```python
from build123d import *
from build123d.topology import SkipClean

# Parameters (mm, degrees)
SKETCH1_W            = 220
SKETCH1_H            = 40
SKETCH1_R            = 6
SKETCH1_R_2          = 1.7
SKETCH1_R_3          = 11
BOSS_EXTRUDE1_DEPTH  = 10
BOSS_EXTRUDE3_START  = -20
SKETCH3_R            = 9.05
SKETCH3_R_2          = 6
BOSS_EXTRUDE3_DEPTH  = 20
SKETCH4_W            = 50
SKETCH4_H            = 65
BOSS_EXTRUDE4_DEPTH  = 10
SKETCH5_W            = 57.5
SKETCH5_H            = 8.5
BOSS_EXTRUDE5_DEPTH  = 20
CUT_EXTRUDE3_START   = -40
SKETCH7_W            = 23
SKETCH7_H            = 15.765385727
CUT_EXTRUDE3_DEPTH   = 40
SKETCH11_W           = 10
SKETCH11_H           = 20
BOSS_EXTRUDE6_DEPTH  = 10
SKETCH12_W           = 10
SKETCH12_H           = 20
BOSS_EXTRUDE7_DEPTH  = 10
FILLET2_R            = 3
FILLET3_R            = 10
BOSS_EXTRUDE8_START  = 10
BOSS_EXTRUDE8_DEPTH  = 10
SKETCH20_R           = 2.15
CUT_EXTRUDE11_DEPTH  = 277
SKETCH19_R           = 2.15
CUT_EXTRUDE12_DEPTH  = 270
BOSS_EXTRUDE9_DEPTH  = 10
SKETCH22_W           = 40
SKETCH22_H           = 40
BOSS_EXTRUDE10_DEPTH = 31.75
SKETCH23_W           = 30.8
SKETCH23_H           = 25.6
CUT_EXTRUDE13_DEPTH  = 263.144
SKETCH24_R           = 4.65
CUT_EXTRUDE14_DEPTH  = 48.144
FILLET4_R            = 3
SKETCH25_R           = 1.7
CUT_EXTRUDE16_DEPTH  = 60.144


with BuildPart() as part:
    # Sketch1 → Boss-Extrude1 (new body)
    with BuildSketch(Plane.XY):
        with Locations((1.5, 0)):
            Rectangle(SKETCH1_W, SKETCH1_H)
        with Locations((99, 0)):
            Circle(SKETCH1_R, mode=Mode.SUBTRACT)
        with Locations((-96, 0)):
            Circle(SKETCH1_R, mode=Mode.SUBTRACT)
        with Locations((-15.5, 15.5)):
            Circle(SKETCH1_R_2, mode=Mode.SUBTRACT)
        with Locations((15.5, 15.5)):
            Circle(SKETCH1_R_2, mode=Mode.SUBTRACT)
        Circle(SKETCH1_R_3, mode=Mode.SUBTRACT)
        with Locations((-15.5, -15.5)):
            Circle(SKETCH1_R_2, mode=Mode.SUBTRACT)
        with Locations((15.5, -15.5)):
            Circle(SKETCH1_R_2, mode=Mode.SUBTRACT)
        with Locations((75, 0)):
            Circle(SKETCH1_R_3, mode=Mode.SUBTRACT)
        with Locations((59.5, 15.5)):
            Circle(SKETCH1_R_2, mode=Mode.SUBTRACT)
        with Locations((59.5, -15.5)):
            Circle(SKETCH1_R_2, mode=Mode.SUBTRACT)
        with Locations((90.5, 15.5)):
            Circle(SKETCH1_R_2, mode=Mode.SUBTRACT)
        with Locations((90.5, -15.5)):
            Circle(SKETCH1_R_2, mode=Mode.SUBTRACT)
    extrude(amount=BOSS_EXTRUDE1_DEPTH)

    # Sketch3 → Boss-Extrude3 (add)
    # profile 1 of 2: a face of its own
    with BuildSketch(Plane.XY.offset(10).offset(BOSS_EXTRUDE3_START)):
        with Locations((-96, 0)):
            Circle(SKETCH3_R)
        with Locations((-96, 0)):
            Circle(SKETCH3_R_2, mode=Mode.SUBTRACT)
    # profile 2 of 2: a face of its own
    with BuildSketch(Plane.XY.offset(10).offset(BOSS_EXTRUDE3_START)):
        with Locations((99, 0)):
            Circle(SKETCH3_R)
        with Locations((99, 0)):
            Circle(SKETCH3_R_2, mode=Mode.SUBTRACT)
    extrude(amount=BOSS_EXTRUDE3_DEPTH)

    # Sketch4 → Boss-Extrude4 (add)
    with BuildSketch(Plane(origin=(111.5, 0, 0), x_dir=(0, 0, -1), z_dir=(1, 0, 0))):
        with Locations((15, 0)):
            Rectangle(SKETCH4_W, SKETCH4_H)
    extrude(amount=BOSS_EXTRUDE4_DEPTH)

    # Sketch5 → Boss-Extrude5 (add)
    with BuildSketch(Plane(origin=(0, 0, 0), x_dir=(-1, 0, 0), z_dir=(0, 0, -1))):
        with Locations((-82.75, 15.75)):
            Rectangle(SKETCH5_W, SKETCH5_H)
        with Locations((-82.75, -15.75)):
            Rectangle(SKETCH5_W, SKETCH5_H)
    extrude(amount=BOSS_EXTRUDE5_DEPTH)

    # Sketch7 → Cut-Extrude3 (cut)
    with BuildSketch(Plane(origin=(0, 20, 0), x_dir=(1, 0, 0), z_dir=(0, 1, 0)).offset(CUT_EXTRUDE3_START)):
        with Locations((72.5, 7.882692864)):
            Rectangle(SKETCH7_W, SKETCH7_H)
    extrude(amount=CUT_EXTRUDE3_DEPTH, mode=Mode.SUBTRACT)

    # Sketch11 → Boss-Extrude6 (add)
    with BuildSketch(Plane(origin=(0, 32.5, 0), x_dir=(1, 0, 0), z_dir=(0, 1, 0))):
        with Locations((116.5, 30)):
            Rectangle(SKETCH11_W, SKETCH11_H)
    extrude(amount=BOSS_EXTRUDE6_DEPTH)

    # Sketch12 → Boss-Extrude7 (add)
    with BuildSketch(Plane.XZ.offset(32.5)):
        with Locations((116.5, -30)):
            Rectangle(SKETCH12_W, SKETCH12_H)
    extrude(amount=BOSS_EXTRUDE7_DEPTH)

    # Fillet2
    # the kernel refuses this fillet: 3 mm, written as the material it adds along each edge
    with BuildSketch(Plane(origin=(121.5, -32.5, -20), x_dir=(0, 0, 1), z_dir=(-1, 0, 0))) as fillet2_piece_1:
        with BuildLine():
            CenterArc((FILLET2_R, -FILLET2_R), FILLET2_R, 90, 90)
            Line((0, -FILLET2_R), (0, 0))
            Line((0, 0), (FILLET2_R, 0))
        make_face()
    extrude(amount=10)
    with BuildSketch(Plane(origin=(111.5, 32.5, -20), x_dir=(0, 1, 0), z_dir=(1, 0, 0))) as fillet2_piece_2:
        with BuildLine():
            CenterArc((FILLET2_R, FILLET2_R), FILLET2_R, 180, 90)
            Line((0, FILLET2_R), (0, 0))
            Line((0, 0), (FILLET2_R, 0))
        make_face()
    extrude(amount=10)
    with BuildSketch(Plane(origin=(84, 11.5, -15.765385727), x_dir=(0, 0, 1), z_dir=(0, 1, 0)), Plane(origin=(61, 11.5, -15.765385727), x_dir=(1, 0, 0), z_dir=(0, 1, 0)), Plane(origin=(84, 11.5, 0), x_dir=(-1, 0, 0), z_dir=(0, 1, 0)), Plane(origin=(84, -20, 0), x_dir=(-1, 0, 0), z_dir=(0, 1, 0))) as fillet2_piece_3:
        with BuildLine():
            CenterArc((FILLET2_R, -FILLET2_R), FILLET2_R, 90, 90)
            Line((0, -FILLET2_R), (0, 0))
            Line((0, 0), (FILLET2_R, 0))
        make_face()
    extrude(amount=8.5)
    with BuildSketch(Plane(origin=(61, 11.5, 0), x_dir=(1, 0, 0), z_dir=(0, 1, 0))) as fillet2_piece_4_section:
        with BuildLine():
            CenterArc((FILLET2_R, FILLET2_R), FILLET2_R, 180, 90)
            Line((0, FILLET2_R), (0, 0))
            Line((0, 0), (FILLET2_R, 0))
        make_face()
    fillet2_piece_4 = extrude(amount=10.7, mode=Mode.PRIVATE)
    fillet2_piece_4 = fillet2_piece_4 - Plane(origin=(59.5, 15.5, -0.653390462), x_dir=(1, 0, 0), z_dir=(0, 0, -1)) * Cylinder(1.7, 34, mode=Mode.PRIVATE)
    fillet2_piece_4 = split(fillet2_piece_4, bisect_by=Plane(origin=(61.689155884, 20, -0.653390462), z_dir=(0, -1, 0)), keep=Keep.TOP, mode=Mode.PRIVATE)
    add(fillet2_piece_4)
    with BuildSketch(Plane(origin=(84, -20, -15.765385727), x_dir=(-1, 0, 0), z_dir=(0, 1, 0))) as fillet2_piece_5:
        with BuildLine():
            CenterArc((FILLET2_R, FILLET2_R), FILLET2_R, 180, 90)
            Line((0, FILLET2_R), (0, 0))
            Line((0, 0), (FILLET2_R, 0))
        make_face()
    extrude(amount=8.5)
    # the kernel refuses this fillet: 3 mm, written as the material it takes off along each edge
    with BuildSketch(Plane(origin=(104, -32.5, 10), x_dir=(0, 0, -1), z_dir=(1, 0, 0)), Plane(origin=(129, -42.5, -20), x_dir=(0, 1, 0), z_dir=(-1, 0, 0)), Plane(origin=(129, 42.5, -40), x_dir=(0, -1, 0), z_dir=(-1, 0, 0))) as fillet2_2_piece_1:
        with BuildLine():
            CenterArc((FILLET2_R, FILLET2_R), FILLET2_R, 180, 90)
            Line((0, FILLET2_R), (0, 0))
            Line((0, 0), (FILLET2_R, 0))
        make_face()
    extrude(amount=25, mode=Mode.SUBTRACT)
    with BuildSketch(Plane(origin=(104, -42.5, -40), x_dir=(0, 0, 1), z_dir=(1, 0, 0)), Plane(origin=(104, 32.5, 10), x_dir=(0, 0, -1), z_dir=(1, 0, 0)), Plane(origin=(104, 42.5, -20), x_dir=(0, 0, -1), z_dir=(1, 0, 0))) as fillet2_2_piece_2:
        with BuildLine():
            CenterArc((FILLET2_R, -FILLET2_R), FILLET2_R, 90, 90)
            Line((0, -FILLET2_R), (0, 0))
            Line((0, 0), (FILLET2_R, 0))
        make_face()
    extrude(amount=25, mode=Mode.SUBTRACT)

    # Fillet3
    fillet3_edges = [part.edges().sort_by_distance(p)[0] for p in [
        (111.5, 15.75, -20),
        (111.5, -15.75, -20),
    ]]
    fillet(fillet3_edges, radius=FILLET3_R)

    # Sketch13 → Boss-Extrude8 (add)
    with BuildSketch(Plane.ZY.offset(108.5).offset(BOSS_EXTRUDE8_START)):
        with BuildLine():
            Line((10, 29.5), (10, -29.5))
            ThreePointArc((10, -29.5), (9.121320344, -31.621320344), (7, -32.5))
            Line((7, -32.5), (-17, -32.5))
            ThreePointArc((-17, -32.5), (-19.121320344, -33.378679656), (-20, -35.5))
            Line((-20, -35.5), (-20, -39.5))
            ThreePointArc((-20, -39.5), (-20.878679656, -41.621320344), (-23, -42.5))
            Line((-23, -42.5), (-37, -42.5))
            ThreePointArc((-37, -42.5), (-39.121320344, -41.621320344), (-40, -39.5))
            Line((-40, -39.5), (-40, 39.5))
            ThreePointArc((-40, 39.5), (-39.121320344, 41.621320344), (-37, 42.5))
            Line((-37, 42.5), (-23, 42.5))
            ThreePointArc((-23, 42.5), (-20.878679656, 41.621320344), (-20, 39.5))
            Line((-20, 39.5), (-20, 35.5))
            ThreePointArc((-20, 35.5), (-19.121320344, 33.378679656), (-17, 32.5))
            Line((-17, 32.5), (7, 32.5))
            ThreePointArc((7, 32.5), (9.121320344, 31.621320344), (10, 29.5))
        make_face()
    extrude(amount=-BOSS_EXTRUDE8_DEPTH)

    # Sketch20 → Cut-Extrude11 (cut)
    with BuildSketch(Plane.ZY.offset(118.5)):
        with Locations((-31, 31.5)):
            Circle(SKETCH20_R)
    extrude(amount=-CUT_EXTRUDE11_DEPTH, mode=Mode.SUBTRACT)

    # Sketch19 → Cut-Extrude12 (cut)
    with BuildSketch(Plane.ZY.offset(118.5)):
        with Locations((-31, -31.5)):
            Circle(SKETCH19_R)
    extrude(amount=-CUT_EXTRUDE12_DEPTH, mode=Mode.SUBTRACT)

    # Sketch16 → Boss-Extrude9 (add)
    with BuildSketch(Plane.XY.offset(10)):
        with BuildLine():
            Line((-98.5, 84), (-118.5, 84))
            Line((-118.5, 84), (-118.5, 29.5))
            Line((-118.5, 29.5), (-108.5, 29.5))
            Line((-108.5, 29.5), (-108.5, 20))
            Line((-108.5, 20), (-78.5, 20))
            ThreePointArc((-78.5, 20), (-92.297269835, 26.202730165), (-98.5, 40))
            Line((-98.5, 40), (-98.5, 84))
        make_face()
    boss_extrude9 = extrude(amount=-BOSS_EXTRUDE9_DEPTH)

    # Mirror1: Boss-Extrude9 across plane
    add(boss_extrude9.mirror(Plane(origin=(1.5, 0, 0), x_dir=(0, 0, 1), z_dir=(1, 0, 0))))

    # Sketch22 → Boss-Extrude10 (add)
    with BuildSketch(Plane(origin=(0, 84, 0), x_dir=(1, 0, 0), z_dir=(0, 1, 0))):
        with Locations((101.5, 10)):
            Rectangle(SKETCH22_W, SKETCH22_H)
    boss_extrude10 = extrude(amount=BOSS_EXTRUDE10_DEPTH)

    # Mirror2: Boss-Extrude10 across plane
    add(boss_extrude10.mirror(Plane(origin=(1.5, 0, 0), x_dir=(0, 0, 1), z_dir=(1, 0, 0))))

    # Sketch23 → Cut-Extrude13 (cut)
    with BuildSketch(Plane.ZY.offset(118.5)):
        with Locations((-10, 102.95)):
            Rectangle(SKETCH23_W, SKETCH23_H)
    extrude(amount=-CUT_EXTRUDE13_DEPTH, mode=Mode.SUBTRACT)

    # Sketch24 → Cut-Extrude14 (cut)
    with BuildSketch(Plane.XZ.offset(-84)):
        with Locations((-98.5, -10)):
            Circle(SKETCH24_R)
        with Locations((101.5, -10)):
            Circle(SKETCH24_R)
    extrude(amount=-CUT_EXTRUDE14_DEPTH, mode=Mode.SUBTRACT)

    # Fillet4
    fillet4_edges = [part.edges().sort_by_distance(p)[0] for p in [
        (-98.5, 84, 5),
        (-108.5, 84, 0),
        (111.5, 84, 0),
        (101.5, 84, 5),
        (101.5, 84, -30),
        (-98.5, 84, -30),
    ]]
    fillet(fillet4_edges, radius=FILLET4_R)

    # Sketch25 → Cut-Extrude16 (cut)
    with SkipClean():  # the faces are left unmerged after this step: merging them gives an invalid solid
        with BuildSketch(Plane(origin=(0, 0, -20), x_dir=(-1, 0, 0), z_dir=(0, 0, -1))):
            with Locations((-90.5, 15.5)):
                Circle(SKETCH25_R)
            with Locations((-59.5, 15.5)):
                Circle(SKETCH25_R)
            with Locations((-90.5, -15.5)):
                Circle(SKETCH25_R)
            with Locations((-59.5, -15.5)):
                Circle(SKETCH25_R)
        extrude(amount=-CUT_EXTRUDE16_DEPTH, mode=Mode.SUBTRACT)


solid = part.part
```
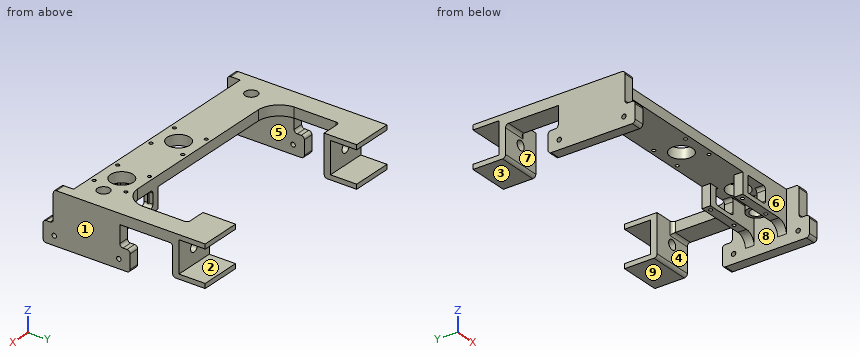
Build history of the part. All positions in model axes, mm. Face numbers are marked on the shaded views. A direction names the side the tool comes from. Give positions to 0.01 mm unless a question says otherwise; leave off trailing zeros. Loops run counter-clockwise (first coordinate to the right, second up) from the corner with the lowest first, then second, coordinate; pieces in that order, holes last. Notation, with made-up numbers: (28, -17.5) -> (49, -17.5) arc R24 cw to (49, 8.5) -> close; hole circle Ø1 at (0, 62.5). An arc over 180 degrees is marked (long way). One line per question, with ' | ' between items. Start each with the question number.
1) 3-axis set-ups, long thin cutter, end or side, ignore diameter. For the marked faces 1, 2, 3, 4 and 5: which of +Z, -Z, +X, -X, +Y, -Y reach the whole face in a straight line?
2) Pin check, flat tips, straight feed: pin 1 (11 mm diameter, centred on x = 99, y = 0, fed in from -Z); pin 2 (5 mm diameter, centred on x = -79, z = -13, fed in from -Y); pin 3 (8 mm diameter, centred on x = -111, z = -7.5, fed in from +Y); pin 4 (14.5 mm diameter, centred on x = 97, y = -3.5, fed in from -Z). Stop position of each tip, or through.
3) Two-plate mould, pull along Y, no slides. Class the marked faces 6, 7, 8 and 9: released by +Y, released by -Y, zero draft, split by the parting line, or undercut.
4) Cut at B-B (y = 45). Give the cut face in (x, z), plus the area to 3 significant figures.
5) Probe L1, parallel to Y at x = 93, z = -19; L2, parallel to X at y = 85, z = -4; L3, parallel to X at y = -4.5, z = -31. List the from-to ranges inside material, lowest first.
6) Cut at A-A (x = 75). Give the cut face in (y, z), plus the area to 3 significant figures.
7) Cut at C-C (x = -2). Give the cut face in (y, z).
Return value:
1) face 1: +Z, -Z, +X, +Y, -Y | face 2: +X, -X, +Y | face 3: -Z, +X, -X, +Y | face 4: -Z | face 5: -Z, -Y
2) pin 1: through | pin 2: y = 84 | pin 3: y = 90.15 | pin 4: z = -10
3) face 6: released by -Y | face 7: undercut | face 8: undercut | face 9: zero draft
4) outline: (-118.5, 0) -> (-98.5, 0) -> (-98.5, 10) -> (-118.5, 10) -> close; (101.5, 0) -> (121.5, 0) -> (121.5, 10) -> (101.5, 10) -> close | area: 400 mm^2
5) L1: -20 to -11.5, 11.5 to 20, 84 to 90.15 | L2: -118.5 to -78.5, 81.5 to 121.5 | L3: -118.5 to -108.5, 111.5 to 121.5
6) outline: (-20, -20) -> (-11.5, -20) -> (-11.5, -15.77) -> (-20, -15.77) -> close; (-20, 0) -> (-11, 0) -> (-11, 10) -> (-20, 10) -> close; (11, 0) -> (20, 0) -> (20, 10) -> (11, 10) -> close; (11.5, -20) -> (20, -20) -> (20, -15.77) -> (11.5, -15.77) -> close | area: 252 mm^2
7) outline: (-20, 0) -> (-10.82, 0) -> (-10.82, 10) -> (-20, 10) -> close; (10.82, 0) -> (20, 0) -> (20, 10) -> (10.82, 10) -> close
